```python
from build123d import *

# Parameters (mm, degrees)
F0_W     = 50.8
F0_H     = 76.2
F1_DEPTH = 3.0988


with BuildPart() as f1:
    # F0 (on Top) → F1 (new body)
    with BuildSketch(Plane.XY):
        Polygon((44.45, 50.8), (-44.45, 50.8), (-44.45, 44.45), (-47.5742, 44.45), (-47.5742, 31.75), (-44.45, 31.75), (-44.45, 6.35), (-47.5742, 6.35), (-47.5742, -6.35), (-44.45, -6.35), (-44.45, -31.75), (-47.5742, -31.75), (-47.5742, -44.45), (-44.45, -44.45), (-44.45, -50.8), (44.45, -50.8), (44.45, -44.45), (47.5742, -44.45), (47.5742, -31.75), (44.45, -31.75), (44.45, -6.35), (47.5742, -6.35), (47.5742, 6.35), (44.45, 6.35), (44.45, 31.75), (47.5742, 31.75), (47.5742, 44.45), (44.45, 44.45), align=None)
        Rectangle(F0_W, F0_H, mode=Mode.SUBTRACT)
    extrude(amount=F1_DEPTH)


solid = f1.part
```
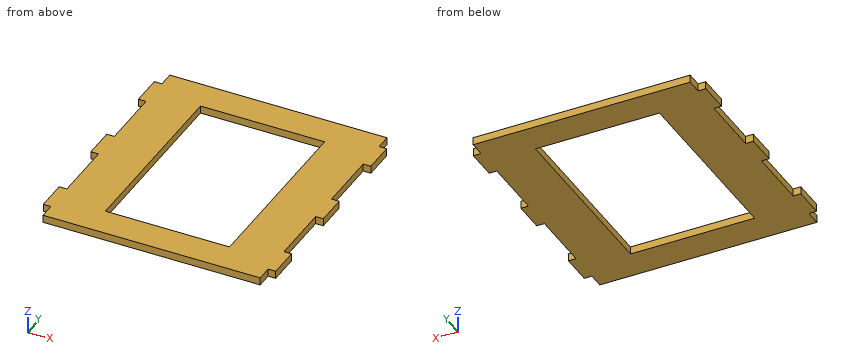
Source: CAD feature listing. Evaluate the final solid. Frame: model axes, mm. Round coordinates to 2 decimals unless told otherwise and drop trailing zeros. Loops run counter-clockwise (first coordinate to the right, second up) from the corner with the lowest first, then second, coordinate; pieces in that order, holes last.
(1) Section query A-A (y = 0.5). Output: boundary loops of the cut face in (x, z), and give its area (3 significant figures).
From the geometry:
outline: (-47.57, 0) - (-25.4, 0) - (-25.4, 3.1) - (-47.57, 3.1) - close; (25.4, 0) - (47.57, 0) - (47.57, 3.1) - (25.4, 3.1) - close
area: 137 mm2
(2) Material intervals for probe 1 along X at (y, z) = (-21, 0.8); probe 2 along X at (y, z) = (-2.5, 1.55); probe 3 along Y at (x, z) = (20, 2.8), sorted ascending.
From the geometry:
probe 1: x = -44.45 to -25.4, 25.4 to 44.45
probe 2: x = -47.57 to -25.4, 25.4 to 47.57
probe 3: y = -50.8 to -38.1, 38.1 to 50.8
(3) Section query B-B (x = 15). Output: boundary loops of the cut face in (y, z).
From the geometry:
outline: (-50.8, 0) - (-38.1, 0) - (-38.1, 3.1) - (-50.8, 3.1) - close; (38.1, 0) - (50.8, 0) - (50.8, 3.1) - (38.1, 3.1) - close
(4) Contact query for flat-ended pins moving along their axis: pin 1 Ø0.9 at (x, z) = (-46.5, 2) entering from -Y; pin 2 Ø1.5 at (y, z) = (24.5, 2.5) entering from -X; pin 3 Ø1.5 at (y, z) = (-23.5, 1) entering from +X. Output: stop coordinate, or through.
From the geometry:
pin 1: stops at y = -44.45
pin 2: stops at x = -44.45
pin 3: stops at x = 44.45
